Study the drawing (mm; zero at the part's minimum x, y, z) and answer. A direction names the side the tool comes from. Give positions to 0.01 mm unless a question says otherwise; leave off trailing zeros. Order: outer loops, then holes, each group sorted by start corner. A loop starts at its lowest first (then second) coordinate and runs counter-clockwise, first axis right, second up. Notation, with made-up numbers: (39, 5.5) - (94, 5.5) arc R16 ccw to (94, 11.5) - close; hole circle Ø9 at (-22.5, -4.5). An arc over 180 degrees is marked (long way). Return JSON: item names as keys, results as strings.
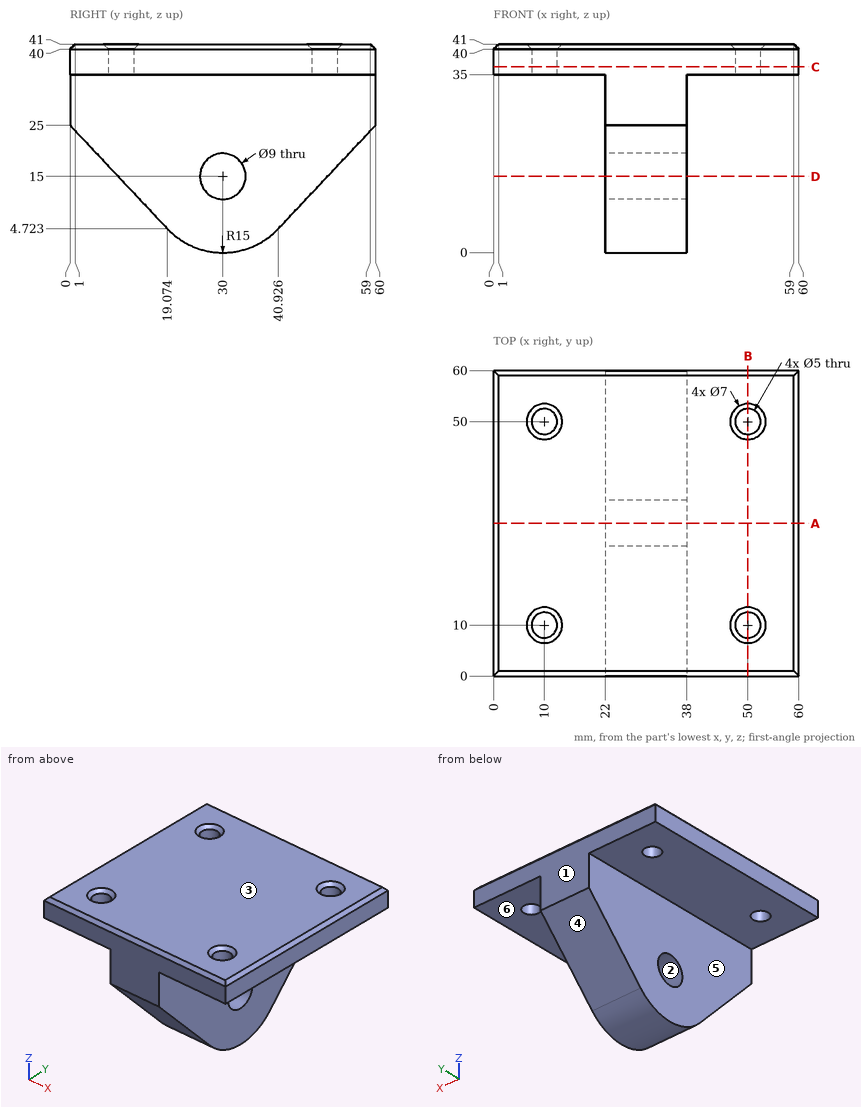
Q1. Determine the mould class of the marked faces 1, 2 and 3 for opening direction Z: released by +Z, released by -Z, zero draft, split by the parting line, or undercut.
Values:
{"face 1": "zero draft", "face 2": "undercut", "face 3": "released by +Z"}
Q2. A cutting plane is placed at A-A (y = 30). Write down the section's boundary in (x, z), and give its area (3 significant figures).
Values:
{"outline": "(0, 35) - (22, 35) - (22, 19.5) - (38, 19.5) - (38, 35) - (60, 35) - (60, 40) - (59, 41) - (1, 41) - (0, 40) - close; (22, 0) - (38, 0) - (38, 10.5) - (22, 10.5) - close", "area": "775 mm²"}
Q3. A cutting plane is placed at B-B (x = 50). Write down the section's boundary in (y, z), and give its area (3 significant figures).
Values:
{"outline": "(0, 35) - (7.5, 35) - (7.5, 40) - (6.5, 41) - (1, 41) - (0, 40) - close; (12.5, 35) - (47.5, 35) - (47.5, 40) - (46.5, 41) - (13.5, 41) - (12.5, 40) - close; (52.5, 35) - (60, 35) - (60, 40) - (59, 41) - (53.5, 41) - (52.5, 40) - close", "area": "297 mm²"}
Q4. A cutting plane is placed at C-C (z = 36.5). Write down the section's boundary in (x, y), and give its area (3 significant figures).
Values:
{"outline": "(0, 0) - (60, 0) - (60, 60) - (0, 60) - close; hole circle Ø5 at (10, 10); hole circle Ø5 at (10, 50); hole circle Ø5 at (50, 10); hole circle Ø5 at (50, 50)", "area": "3,520 mm²"}
Q5. Given pin 1 (1.5 mm diameter, centred on x = 42, y = 47.5, fed in from -Z); pin 2 (10.5 mm diameter, centred on y = 31.5, z = 13.5, fed in from +X); pin 3 (6 mm diameter, centred on x = 50, y = 10, fed in from +Z), each flat-ended and moving along its own axis, determine where each tip first touches the part or whether it passes through.
Values:
{"pin 1": "stops at z = 35", "pin 2": "stops at x = 38", "pin 3": "stops at z = 40.5"}
Q6. A cutting plane is placed at D-D (z = 15). Write down the section's boundary in (x, y), and give its area (3 significant figures).
Values:
{"outline": "(22, 9.41) - (38, 9.41) - (38, 25.5) - (22, 25.5) - close; (22, 34.5) - (38, 34.5) - (38, 50.59) - (22, 50.59) - close", "area": "515 mm²"}
Q7. Consider L1, parallel to Y at x = 10, z = 38; L2, parallel to Z at x = 54, y = 52; L3, parallel to X at y = 19.5, z = 19.5. Determine where each line is inside the solid, lowest interval first.
Values:
{"L1": "y = 0 to 7.5, 12.5 to 47.5, 52.5 to 60", "L2": "z = 35 to 41", "L3": "x = 22 to 38"}
Q8. For the marked faces 4, 5 and 6, determine the directions among +Z, -Z, +X, -X, +Y, -Y from which every point of the face is accessible in a straight line to the end or side of a thin tool.
Values:
{"face 4": "-Z, +X, -X, +Y", "face 5": "-Z, -X, +Y, -Y", "face 6": "-Z, +X, +Y, -Y"}
